Design review of the part built by this model. Coordinates are the model's own, in mm. Face numbers are marked on the shaded views. A direction names the side the tool comes from. Give positions to 0.01 mm unless a question says otherwise; leave off trailing zeros. Loops run counter-clockwise (first coordinate to the right, second up) from the corner with the lowest first, then second, coordinate; pieces in that order, holes last. Notation, with made-up numbers: (-5, 17.25) -> (47, 17.25) arc R17 cw to (47, 33.25) -> close; hole circle Ø6 at (8, 86). An arc over 180 degrees is marked (long way). Use a Markdown table: item, result. Add a question column.
1. Add section B-B (x = 11.5). State the section outline as (y, z) points (3 decimals), and give its area (3 significant figures).
2. For the marked faces 1 and 2, list the 3-axis set-ups (+Z, -Z, +X, -X, +Y, -Y) from which the entire face can be reached by the end or side of a thin tool; tool diameter is ignored.
3. For pin 1 Ø8 at (y, z) = (14, -1.5) entering from +X, flat-tipped, find the tip position at first contact; note if it passes through.
4. To check wall thickness, follow line 1 (Y direction, x = -116.5, z = -6); line 2 (Z direction, x = 154.5, y = 16). State the ranges of each line that lie inside material, in increasing order.
5. Draft analysis for pull direction Z (two halves, no side actions). For the marked faces 3, 4 and 5, state which applies: pulls with the +Z half, pulls with the -Z half, needs draft (parallel to the pull), parting line crosses it, or undercut.
6. Add section A-A (y = 2.5). State the section outline as (x, z) points, and give its area (3 significant figures).
7. Add section C-C (z = 2.5). State the section outline as (x, y) points, and give its area (3 significant figures).
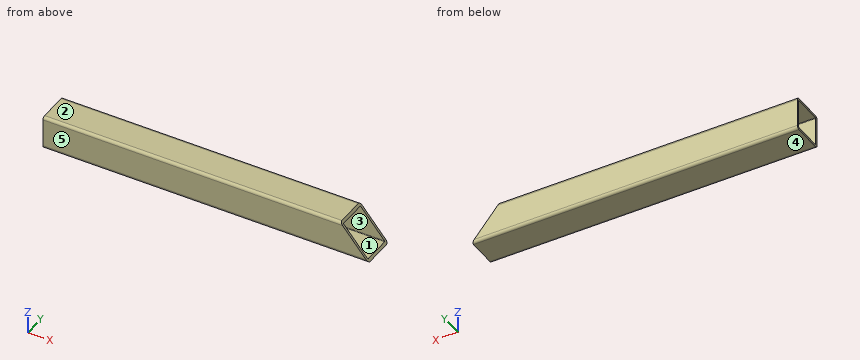
```python
from build123d import *

# Parameters (mm, degrees)
EXTRUDE_THIN1_DEPTH     = 184.15
CUT_EXTRUDE1_DEPTH      = 1
CUT_EXTRUDE1_DEPTH_BACK = 39.1


with BuildPart() as part:
    # Sketch1 → Extrude-Thin1 (new body, symmetric)
    with BuildSketch(Plane(origin=(0, 0, 0), x_dir=(0, 0, -1), z_dir=(1, 0, 0))):
        with BuildLine():
            Line((-15.875, 19.05), (15.875, 19.05))
            ThreePointArc((15.875, 19.05), (18.12006403, 18.12006403), (19.05, 15.875))
            Line((19.05, 15.875), (19.05, -15.875))
            ThreePointArc((19.05, -15.875), (18.12006403, -18.12006403), (15.875, -19.05))
            Line((15.875, -19.05), (-15.875, -19.05))
            ThreePointArc((-15.875, -19.05), (-18.12006403, -18.12006403), (-19.05, -15.875))
            Line((-19.05, -15.875), (-19.05, 15.875))
            ThreePointArc((-19.05, 15.875), (-18.12006403, 18.12006403), (-15.875, 19.05))
        make_face()
        with BuildLine():
            Line((-15.875, 16.51), (15.875, 16.51))
            ThreePointArc((15.875, 16.51), (16.324012806, 16.324012806), (16.51, 15.875))
            Line((16.51, 15.875), (16.51, -15.875))
            ThreePointArc((16.51, -15.875), (16.324012806, -16.324012806), (15.875, -16.51))
            Line((15.875, -16.51), (-15.875, -16.51))
            ThreePointArc((-15.875, -16.51), (-16.324012806, -16.324012806), (-16.51, -15.875))
            Line((-16.51, -15.875), (-16.51, 15.875))
            ThreePointArc((-16.51, 15.875), (-16.324012806, 16.324012806), (-15.875, 16.51))
        make_face(mode=Mode.SUBTRACT)
    extrude(amount=EXTRUDE_THIN1_DEPTH, both=True)

    # Sketch3 → Cut-Extrude1 (cut, two sides)
    with BuildSketch(Plane(origin=(0, 19.05, 0), x_dir=(1, 0, 0), z_dir=(0, 1, 0))) as cut_extrude1_sk:
        Polygon((666.581957194, 593.990018168), (184.15, 19.05), (152.180304052, -19.05), (-330.251653142, -593.990018168), (819.628383194, -1558.853932556), (1816.46199353, -370.87389622), align=None)
    extrude(amount=CUT_EXTRUDE1_DEPTH, mode=Mode.SUBTRACT)
    extrude(cut_extrude1_sk.sketch, amount=-CUT_EXTRUDE1_DEPTH_BACK, mode=Mode.SUBTRACT)


solid = part.part
```
Taken from the geometry:
| question | item | result |
|---|---|---|
| 1 | outline | (-19.05, -15.875) arc R3.175 ccw to (-15.875, -19.05) -> (15.875, -19.05) arc R3.175 ccw to (19.05, -15.875) -> (19.05, 15.875) arc R3.175 ccw to (15.875, 19.05) -> (-15.875, 19.05) arc R3.175 ccw to (-19.05, 15.875) -> close; hole (-16.51, -15.875) arc R0.635 ccw to (-15.875, -16.51) -> (15.875, -16.51) arc R0.635 ccw to (16.51, -15.875) -> (16.51, 15.875) arc R0.635 ccw to (15.875, 16.51) -> (-15.875, 16.51) arc R0.635 ccw to (-16.51, 15.875) -> close |
| 1 | area | 353 mm^2 |
| 2 | face 1 | +X, -X |
| 2 | face 2 | +Z, +X, -X, +Y, -Y |
| 3 | pin 1 | stops at x = 172.04 |
| 4 | line 1 | y = -19.05 to -16.51, 16.51 to 19.05 |
| 4 | line 2 | z = -19.05 to -16.5 |
| 5 | face 3 | undercut |
| 5 | face 4 | pulls with the -Z half |
| 5 | face 5 | needs draft |
| 6 | outline | (-184.15, -19.05) -> (184.15, -19.05) -> (182.02, -16.51) -> (-184.15, -16.51) -> close; (-184.15, 16.51) -> (154.31, 16.51) -> (152.18, 19.05) -> (-184.15, 19.05) -> close |
| 6 | area | 1,790 mm^2 |
| 7 | outline | (-184.15, -19.05) -> (166.07, -19.05) -> (166.07, -16.51) -> (-184.15, -16.51) -> close; (-184.15, 16.51) -> (166.07, 16.51) -> (166.07, 19.05) -> (-184.15, 19.05) -> close |
| 7 | area | 1,780 mm^2 |
